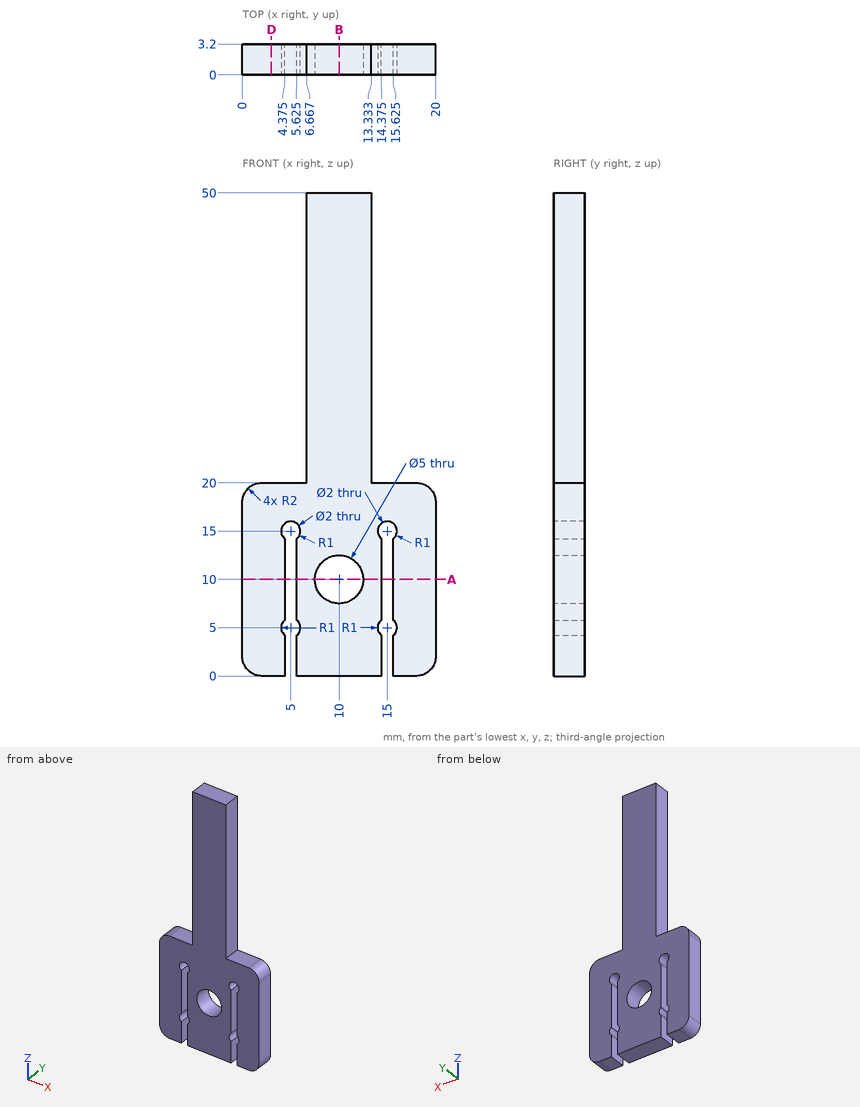
Could you check a few things on this drawing? It's one solid part, dimensions in mm from its lowest x, y, z. Round coordinates to 2 decimals unless told otherwise and drop trailing zeros. Order: outer loops, then holes, each group sorted by start corner. A loop starts at its lowest first (then second) coordinate and runs counter-clockwise, first axis right, second up.
(1) Imagine slicing it at B-B (x = 10). Write out the boundary of the cut face in (y, z).
Response values:
outline: (0, 0) - (3.2, 0) - (3.2, 7.5) - (0, 7.5) - close; (0, 12.5) - (3.2, 12.5) - (3.2, 50) - (0, 50) - close
(2) Imagine slicing it at D-D (x = 3). Write out the boundary of the cut face in (y, z).
Response values:
outline: (0, 0) - (3.2, 0) - (3.2, 20) - (0, 20) - close
(3) Please list where these lines run through material, in increasing order: line 1 along X through (y, z) = (1.2, 10) (1 decimal); line 2 along X through (y, z) = (1.45, 15); line 3 along Z through (x, y) = (15.75, 2.15).
Response values:
line 1: x = 0 to 4.4, 5.6 to 7.5, 12.5 to 14.4, 15.6 to 20
line 2: x = 0 to 4, 6 to 14, 16 to 20
line 3: z = 0 to 4.34, 5.66 to 14.34, 15.66 to 20
(4) Imagine slicing it at A-A (z = 10). Write out the boundary of the cut face in (x, y) (1 decimal), plus the area to 3 significant figures.
Response values:
outline: (0, 0) - (4.4, 0) - (4.4, 3.2) - (0, 3.2) - close; (5.6, 0) - (7.5, 0) - (7.5, 3.2) - (5.6, 3.2) - close; (12.5, 0) - (14.4, 0) - (14.4, 3.2) - (12.5, 3.2) - close; (15.6, 0) - (20, 0) - (20, 3.2) - (15.6, 3.2) - close
area: 40.0 mm2
(5) I'm going to push flat-ended pins straight in: pin 1 (1 mm diameter, centred on y = 2.5, z = 27.5, fed in from +X); pin 2 (1 mm diameter, centred on x = 14.5, y = 2.5, fed in from +Z); pin 3 (1 mm diameter, centred on y = 1.5, z = 33.5, fed in from -X); pin 4 (4.5 mm diameter, centred on x = 10, z = 10, fed in from -Y). Where does each tip first touch, or does it pass through?
Response values:
pin 1: stops at x = 13.33
pin 2: stops at z = 20
pin 3: stops at x = 6.67
pin 4: passes through
